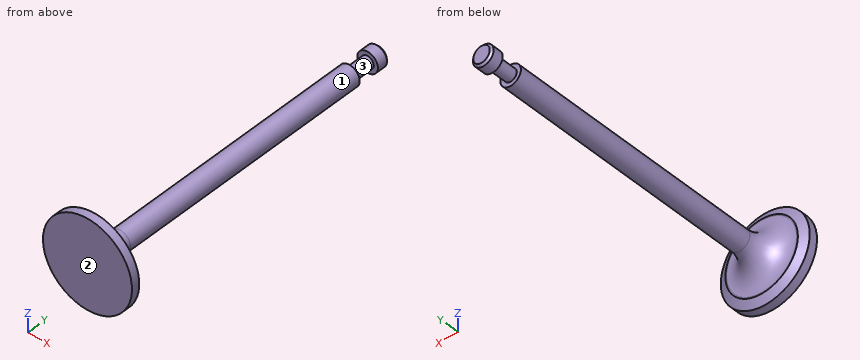
```python
from build123d import *

# Parameters (mm, degrees)
FILLET1_R      = 6
CHAMFER1_SIZE  = 0.5
CHAMFER2_SIZE  = 2
CHAMFER2_SIZE2 = 1


with BuildPart() as part:
    # Sketch1 → Revolve1 (revolve)
    with BuildSketch(Plane.XY, mode=Mode.PRIVATE) as revolve1_sk:
        Polygon((0, 0), (0, 80), (2.5, 80), (2.5, 77), (1.5, 77), (1.5, 72), (2.5, 72), (2.5, 3), (10.793050135, 3), (10.793050135, 0), align=None)
    revolve(revolve1_sk.sketch.rotate(Axis((0, 0, 0), (0, 1, 0)), 90), axis=Axis((0, 0, 0), (0, 1, 0)))

    # Fillet1
    fillet1_edges = [part.edges().sort_by_distance(p)[0] for p in [
        (0, 3, 2.5),
    ]]
    fillet(fillet1_edges, radius=FILLET1_R)

    # Chamfer1
    chamfer1_edges = [part.edges().sort_by_distance(p)[0] for p in [
        (0, 80, 2.5),
    ]]
    chamfer(chamfer1_edges, length=CHAMFER1_SIZE)

    # Chamfer2
    chamfer2_edges = [part.edges().sort_by_distance(p)[0] for p in [
        (0, 3, 10.793050135),
    ]]
    chamfer2_side = [part.faces().sort_by_distance(p)[0] for p in [
        (0, 3, 8.805273558),
    ]]
    chamfer(chamfer2_edges, length=CHAMFER2_SIZE, length2=CHAMFER2_SIZE2, reference=chamfer2_side[0])


solid = part.part
```
Geometry check sheet. Reference: the model listing, model coordinates, mm. Face numbers are marked on the shaded views. Round coordinates to 2 decimals unless told otherwise and drop trailing zeros. Loops run counter-clockwise (first coordinate to the right, second up) from the corner with the lowest first, then second, coordinate; pieces in that order, holes last. Notation, with made-up numbers: M 34.5,8 L 65.5,8 A32 cw 65.5,42 Z; hole C 11.25,28 d10. An arc over 180 degrees is marked long. Return JSON: item names as keys, results as strings. Group by question number.
(1) Go/stop test with flat-tipped pins: pin 1 (5 mm diameter, centred on x = -1.5, y = 54.5, fed in from -Z); pin 2 (1.5 mm diameter, centred on y = 33.5, z = 1.5, fed in from +X); pin 3 (4 mm diameter, centred on x = -0.5, z = 8, fed in from +Y); pin 4 (1 mm diameter, centred on x = -7, z = -2, fed in from -Y). Record where each tip stops, or that it passes through.
(2) Scan lines: line 1 along X through (y, z) = (34, 1.5); line 2 along Y through (x, z) = (1.5, -8). Record each from-to range of solid material in increasing order. Write a range as [from, to].
(3) Section check B-B, the plane x = 0. Enter the section's corners in (y, z).
(4) Section check C-C, the plane y = 64. Enter the section's corners in (x, z), and give its area (3 significant figures).
(5) Mould release check, pull along Y, two halves, no side actions. Record for the marked faces 1, 2 and 3: pulls with the +Y half, pulls with the -Y half, needs draft (parallel to the pull), parting line crosses it, or undercut.
(6) Section check A-A, the plane z = 0. Enter the section's corners in (x, y), and give its area (3 significant figures).
Data:
{
 "1": {"pin 1": "z = -2.5", "pin 2": "x = 2.38", "pin 3": "y = 3.54", "pin 4": "y = 0"},
 "2": {"line 1": "[-2, 2]", "line 2": "[0, 3.01]"},
 "3": {"outline": "M 0,-10.79 L 2,-10.79 L 3,-8.79 L 3,-8.5 A6 cw 9,-2.5 L 72,-2.5 L 72,-1.5 L 77,-1.5 L 77,-2.5 L 79.5,-2.5 L 80,-2 L 80,2 L 79.5,2.5 L 77,2.5 L 77,1.5 L 72,1.5 L 72,2.5 L 9,2.5 A6 cw 3,8.5 L 3,8.79 L 2,10.79 L 0,10.79 Z"},
 "4": {"outline": "C 0,0 d5", "area": "19.6 mm²"},
 "5": {"face 1": "needs draft", "face 2": "pulls with the -Y half", "face 3": "undercut"},
 "6": {"outline": "M -10.79,0 L 10.79,0 L 10.79,2 L 8.79,3 L 8.5,3 A6 cw 2.5,9 L 2.5,72 L 1.5,72 L 1.5,77 L 2.5,77 L 2.5,79.5 L 2,80 L -2,80 L -2.5,79.5 L -2.5,77 L -1.5,77 L -1.5,72 L -2.5,72 L -2.5,9 A6 cw -8.5,3 L -8.79,3 L -10.79,2 Z", "area": "453 mm²"}
}
